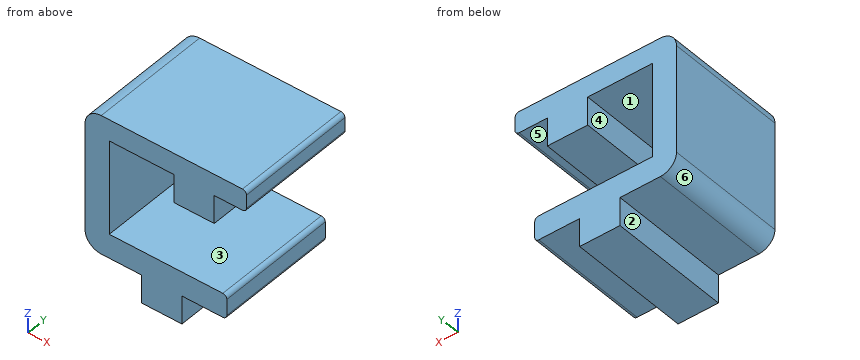
```python
from build123d import *

# Parameters (mm, degrees)
BOSS_EXTRUDE1_DEPTH = 15
SKETCH2_W           = 5
SKETCH2_H           = 15
BOSS_EXTRUDE2_DEPTH = 3.5
SKETCH3_W           = 5
SKETCH3_H           = 15
BOSS_EXTRUDE3_DEPTH = 3.5
FILLET1_R           = 2
FILLET2_R           = 0.5


with BuildPart() as part:
    # Sketch1 → Boss-Extrude1 (new body)
    with BuildSketch(Plane(origin=(0, 0, 0), x_dir=(1, 0, 0), z_dir=(0, 1, 0))):
        Polygon((0, 0), (-20, 0), (-20, 17.325), (-2.435474502, 17.325), (-2.435474502, 14.325), (-17, 14.325), (-17, 2.65), (0, 2.65), align=None)
    extrude(amount=BOSS_EXTRUDE1_DEPTH)

    # Sketch2 → Boss-Extrude2 (add)
    with BuildSketch(Plane(origin=(0, 0, -2.65), x_dir=(-1, 0, 0), z_dir=(0, 0, -1))):
        with Locations((6.5, 7.5)):
            Rectangle(SKETCH2_W, SKETCH2_H)
    extrude(amount=BOSS_EXTRUDE2_DEPTH)

    # Sketch3 → Boss-Extrude3 (add)
    with BuildSketch(Plane(origin=(0, 0, -17.325), x_dir=(-1, 0, 0), z_dir=(0, 0, -1))):
        with Locations((10.5, 7.5)):
            Rectangle(SKETCH3_W, SKETCH3_H)
    extrude(amount=BOSS_EXTRUDE3_DEPTH)

    # Fillet1
    fillet1_edges = [part.edges().sort_by_distance(p)[0] for p in [
        (-20, 7.5, 0),
        (-20, 7.5, -17.325),
    ]]
    fillet(fillet1_edges, radius=FILLET1_R)

    # Fillet2
    fillet2_edges = [part.edges().sort_by_distance(p)[0] for p in [
        (0, 7.5, 0),
        (-2.435474502, 7.5, -17.325),
        (-2.435474502, 7.5, -14.325),
        (0, 7.5, -2.65),
    ]]
    fillet(fillet2_edges, radius=FILLET2_R)


solid = part.part
```
CAD build for the part. Positions are in the model's coordinates, mm. Face numbers are marked on the shaded views. A direction names the side the tool comes from. Give positions to 0.01 mm unless a question says otherwise; leave off trailing zeros. Order: outer loops, then holes, each group sorted by start corner. A loop starts at its lowest first (then second) coordinate and runs counter-clockwise, first axis right, second up.
(1) Tool access for the marked faces 1, 2 and 3: list every direction of +Z, -Z, +X, -X, +Y, -Y with a clear straight run to the whole face (end or side of a thin tool).
(2) Saw through at D-D, the plane z = -10.5. Give the cut face in (x, y).
(3) Drill centre lines: L1, parallel to X at y = 8.5, z = -3; L2, parallel to Z at x = -4.75, y = 8.5 (3 decimals); L3, parallel to Z at x = -3.5, y = 11.5 (3 decimals). Where is each one in solid material? Low to high.
(4) Saw through at B-B, the plane y = 6. Give the cut face in (x, z) (3 decimals), then the cut area to 3 significant figures.
(5) Flat gauge pins, fed straight in: pin 1 (4 mm diameter, centred on y = 6.5, z = -19, fed in from -X); pin 2 (2.5 mm diameter, centred on x = -5, y = 6.5, fed in from -Z) (3 decimals); pin 3 (4 mm diameter, centred on x = -13.5, z = -10, fed in from +Y); pin 4 (6 mm diameter, centred on y = 4.5, z = -17.5, fed in from +X). Where does each tip first touch, or does it go through?
(6) Saw through at C-C, the plane x = -15.5. Give the cut face in (y, z) (3 decimals), then the cut area to 4 significant figures.
(7) Mould opens along X. For the marked faces 4, 5 and 6 say: released by +X, released by -X, zero draft, split by the parting line, or undercut.
(8) Saw through at A-A, the plane x = -5. Give the cut face in (y, z) (3 decimals), then the cut area to 3 significant figures.
Results found:
1. face 1: +Y, -Y
1. face 2: -Z, -X, +Y, -Y
1. face 3: +X, +Y, -Y
2. outline: (-20, 0) - (-17, 0) - (-17, 15) - (-20, 15) - close
3. L1: x = -20 to -17, -9 to -4
3. L2: z = -17.325 to -14.325, -6.15 to 0
3. L3: z = -17.325 to -14.325, -2.65 to 0
4. outline: (-20, -15.325) arc R2 ccw to (-18, -17.325) - (-13, -17.325) - (-13, -20.825) - (-8, -20.825) - (-8, -17.325) - (-2.935, -17.325) arc R0.5 ccw to (-2.435, -16.825) - (-2.435, -14.825) arc R0.5 ccw to (-2.935, -14.325) - (-17, -14.325) - (-17, -2.65) - (-9, -2.65) - (-9, -6.15) - (-4, -6.15) - (-4, -2.65) - (-0.5, -2.65) arc R0.5 ccw to (0, -2.15) - (0, -0.5) arc R0.5 ccw to (-0.5, 0) - (-18, 0) arc R2 ccw to (-20, -2) - close
4. area: 174 mm2
5. pin 1: stops at x = -19.09
5. pin 2: stops at z = -17.325
5. pin 3: passes through
5. pin 4: stops at x = -2.44
6. outline: (0, -17.325) - (15, -17.325) - (15, -14.325) - (0, -14.325) - close; (0, -2.65) - (15, -2.65) - (15, 0) - (0, 0) - close
6. area: 84.75 mm2
7. face 4: undercut
7. face 5: zero draft
7. face 6: released by -X
8. outline: (0, -17.325) - (15, -17.325) - (15, -14.325) - (0, -14.325) - close; (0, -6.15) - (15, -6.15) - (15, 0) - (0, 0) - close
8. area: 137 mm2
